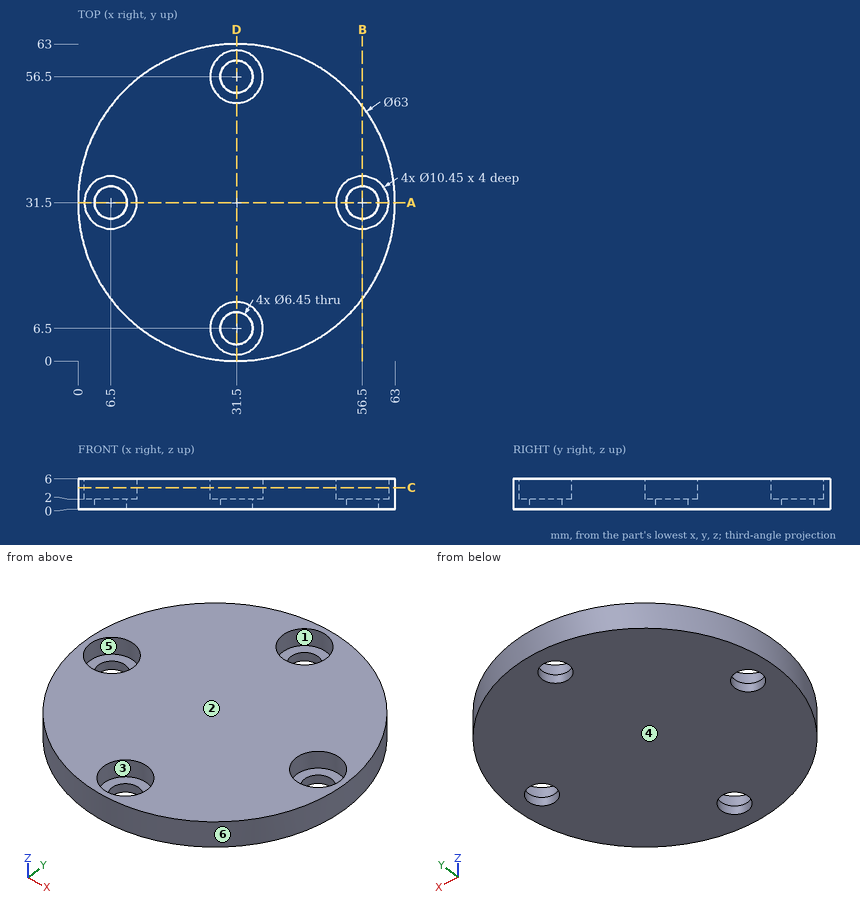
For this review, use the dimensioned drawing (mm, ordinates from the lowest corner) and the shaded views. A direction names the side the tool comes from. Coordinates: 2 decimals unless noted, no trailing zeros. Loops run counter-clockwise (first coordinate to the right, second up) from the corner with the lowest first, then second, coordinate; pieces in that order, holes last. Notation, with made-up numbers: (27, 48) -> (76, 48) arc R19 ccw to (76, 79) -> close; hole circle Ø9 at (1.25, 19.25). An arc over 180 degrees is marked (long way). Use a Markdown table: item, result. Add a question column.
Item 1: We need section C-C, the plane z = 4.3. Write out the cut boundary in (x, y) (3 decimals), and give its area (3 significant figures).
Item 2: Clearance check with flat-ended pins moving along their axes: P1, Ø10.5, axis at x = 31.5, y = 6.5, coming from the -Z side; P2, Ø4, axis at x = 56.5, y = 31.5, coming from the +Z side; P3, Ø1, axis at x = 52, z = 2.5, coming from the -Y side; P4, Ø1, axis at x = 43.5, z = 5, coming from the +Y side. State where each tip first meets the part, or that it passes through.
Item 3: Machinability: for the marked faces 1 and 2, which of the approach directions +Z, -Z, +X, -X, +Y, -Y give a long, thin tool a straight path to every point of the face, cutting with its end or side? Answer none if there is none.
Item 4: We need section B-B, the plane x = 56.5. Write out the cut boundary in (y, z) (3 decimals), and give its area (3 significant figures).
Item 5: The part is to be moulded in two halves that separate along Y. For the marked faces 3, 4, 5 and 6, say which applies: +Y half, -Y half, draft (parallel to the pull), parting line (faces both ways), or undercut.
Item 6: Wall thickness on L1, parallel to Y at x = 31.5, z = 1.5 (3 decimals); L2, parallel to Y at x = 6, z = 3.8; L3, parallel to X at y = 56, z = 3.4: over which ranges is each line inside the solid? List them lowest first. Write a range as from..to.
Item 7: We need section A-A, the plane y = 31.5. Write out the cut boundary in (x, z) (3 decimals).
Numbers:
| question | item | result |
|---|---|---|
| 1 | outline | circle Ø63 at (31.5, 31.5); hole circle Ø10.45 at (6.5, 31.5); hole circle Ø10.45 at (31.5, 6.5); hole circle Ø10.45 at (31.5, 56.5); hole circle Ø10.45 at (56.5, 31.5) |
| 1 | area | 2,770 mm^2 |
| 2 | P1 | stops at z = 0 |
| 2 | P2 | passes through |
| 2 | P3 | stops at y = 7.16 |
| 2 | P4 | stops at y = 60.83 |
| 3 | face 1 | +Z |
| 3 | face 2 | +Z, +X, -X, +Y, -Y |
| 4 | outline | (12.336, 0) -> (28.275, 0) -> (28.275, 2) -> (26.275, 2) -> (26.275, 6) -> (12.336, 6) -> close; (34.725, 0) -> (50.664, 0) -> (50.664, 6) -> (36.725, 6) -> (36.725, 2) -> (34.725, 2) -> close |
| 4 | area | 175 mm^2 |
| 5 | face 3 | undercut |
| 5 | face 4 | draft |
| 5 | face 5 | undercut |
| 5 | face 6 | parting line |
| 6 | L1 | y = 0..3.275, 9.725..53.275, 59.725..63 |
| 6 | L2 | y = 13.01..26.3, 36.7..49.99 |
| 6 | L3 | x = 11.7..26.3, 36.7..51.3 |
| 7 | outline | (0, 0) -> (3.275, 0) -> (3.275, 2) -> (1.275, 2) -> (1.275, 6) -> (0, 6) -> close; (9.725, 0) -> (53.275, 0) -> (53.275, 2) -> (51.275, 2) -> (51.275, 6) -> (11.725, 6) -> (11.725, 2) -> (9.725, 2) -> close; (59.725, 0) -> (63, 0) -> (63, 6) -> (61.725, 6) -> (61.725, 2) -> (59.725, 2) -> close |
